Can you work these out from the model? Positions are in its coordinate system, mm. A direction names the side the tool comes from. Coordinates: 2 decimals unless noted, no trailing zeros. Write each loop counter-clockwise with the first axis right and the second up, starting at its lowest first coordinate (ties: lowest second). Pieces come first, ordered by that corner, then holes. Notation, with made-up numbers: (37, 17) - (86, 17) arc R13 cw to (86, 22) - close; hole circle Ø11 at (-23.5, -5.75). An arc over 180 degrees is marked (long way). Write each question's results on one line, items separated by ' | '. Start each with the question number.
```python
from build123d import *

# Parameters (mm, degrees)
SKETCH1_W              = 25
SKETCH1_H              = 25
SKETCH1_R              = 9.5
ALONGSIDE_WASHER_DEPTH = 2
SKETCH2_W              = 25
SKETCH2_H              = 25
BELOW_WASHER_DEPTH     = 1
SKETCH3_W              = 5
SKETCH3_H              = 25
UPRIGHT_1_DEPTH        = 15.6
SKETCH4_W              = 25
SKETCH4_H              = 1.2
BOSS_EXTRUDE4_DEPTH    = 25
SKETCH5_R              = 2.75
CUT_EXTRUDE1_DEPTH     = 1.2
BOSS_EXTRUDE5_START    = -1.2
SKETCH6_W              = 25
SKETCH6_H              = 25
BOSS_EXTRUDE5_DEPTH    = 6.2
SKETCH7_R              = 3.1
CUT_EXTRUDE2_DEPTH     = 40.930063862
SKETCH8_W              = 25
SKETCH8_H              = 4.2
BOSS_EXTRUDE6_DEPTH    = 37
BOSS_EXTRUDE7_START    = -1
SKETCH9_R              = 1
BOSS_EXTRUDE7_DEPTH    = 1


with BuildPart() as part:
    # Sketch1 → alongside washer (new body)
    with BuildSketch(Plane(origin=(0, 0, 0), x_dir=(1, 0, 0), z_dir=(0, 1, 0))):
        Rectangle(SKETCH1_W, SKETCH1_H)
        with Locations(Location((0, 0, 0), (0, 0, 270))):
            Circle(SKETCH1_R, mode=Mode.SUBTRACT)
    extrude(amount=ALONGSIDE_WASHER_DEPTH)

    # Sketch2 → below washer (add)
    with BuildSketch(Plane.XZ):
        Rectangle(SKETCH2_W, SKETCH2_H)
    extrude(amount=BELOW_WASHER_DEPTH)

    # Sketch3 → upright 1 (add)
    with BuildSketch(Plane.XZ.offset(1)):
        with Locations((-15, 0)):
            Rectangle(SKETCH3_W, SKETCH3_H)
    upright_1 = extrude(amount=-UPRIGHT_1_DEPTH)

    # Sketch4 → Boss-Extrude4 (add)
    with BuildSketch(Plane(origin=(-12.5, 0, 0), x_dir=(0, 0, -1), z_dir=(1, 0, 0))):
        with Locations((0, 8)):
            Rectangle(SKETCH4_W, SKETCH4_H)
    extrude(amount=BOSS_EXTRUDE4_DEPTH)

    # Sketch5 → Cut-Extrude1 (cut)
    with BuildSketch(Plane(origin=(0, 8.6, 0), x_dir=(1, 0, 0), z_dir=(0, 1, 0))):
        with Locations(Location((0, 0, 0), (0, 0, 270))):
            Circle(SKETCH5_R)
    extrude(amount=-CUT_EXTRUDE1_DEPTH, mode=Mode.SUBTRACT)

    # Sketch6 → Boss-Extrude5 (add)
    with BuildSketch(Plane(origin=(0, 8.6, 0), x_dir=(1, 0, 0), z_dir=(0, 1, 0)).offset(BOSS_EXTRUDE5_START)):
        Rectangle(SKETCH6_W, SKETCH6_H)
        Polygon((3.9, 2.25166605), (0, 4.5033321), (-3.9, 2.25166605), (-3.9, -2.25166605), (0, -4.5033321), (3.9, -2.25166605), align=None, mode=Mode.SUBTRACT)
    extrude(amount=BOSS_EXTRUDE5_DEPTH)

    # Mirror1: upright 1 across plane
    add(upright_1.mirror(Plane(origin=(0, 0, 0), x_dir=(0, 0, 1), z_dir=(1, 0, 0))))

    # Sketch7 → Cut-Extrude2 (cut, through all)
    with BuildSketch(Plane(origin=(17.5, 0, 0), x_dir=(0, 0, -1), z_dir=(1, 0, 0))):
        with Locations((0, 5.2)):
            Circle(SKETCH7_R)
    extrude(amount=-CUT_EXTRUDE2_DEPTH, mode=Mode.SUBTRACT)

    # Sketch8 → Boss-Extrude6 (add)
    with BuildSketch(Plane(origin=(12.5, 0, 0), x_dir=(0, 0, -1), z_dir=(1, 0, 0))):
        with Locations((0, 12.5)):
            Rectangle(SKETCH8_W, SKETCH8_H)
    extrude(amount=BOSS_EXTRUDE6_DEPTH)

    # Sketch9 → Boss-Extrude7 (add)
    with BuildSketch(Plane.ZY.offset(-12.5).offset(BOSS_EXTRUDE7_START)):
        with BuildLine():
            ThreePointArc((-2.184032967, 7.4), (-1.191532166, 2.338138526), (3.1, 5.2))
            ThreePointArc((3.1, 5.2), (2.861861474, 6.391532166), (2.184032967, 7.4))
            ThreePointArc((2.184032967, 7.4), (0, 8.3), (-2.184032967, 7.4))
        make_face()
        with Locations((0, 5.2)):
            Circle(SKETCH9_R, mode=Mode.SUBTRACT)
    extrude(amount=BOSS_EXTRUDE7_DEPTH)


solid = part.part
```
Q1. If we section it at C-C (z = 0): Count the separate pieces of the cut face and the enclosed holes in it, then the cut area to 3 significant figures.
Q2. I need wall thicknesses on line 1 along X through (y, z) = (2.25, 2.75); line 2 along Y through (x, z) = (-9, -8); line 3 along Y through (x, z) = (-5.5, 0). Which ranges of each line are inside material? Lowest first, please. Write a range as from..to.
Q3. Thinking about a two-plate mould opening in X: for faces 1 (the face through (13.5, 6, -1)), 2 (the face through (-9, 2, -6)), 3 (the face through (15.528, 4.013, -2.864)), which applies, pulls with the +X half, pulls with the -X half, needs draft (parallel to the pull), parting line crosses it, or undercut?
Q4. If we section it at B-B (x = -7.5): Please give me the cut outline in (y, z).
Q5. For faces 4 (the face through (1.98, 11.06, -3.36)), 5 (the face through (-12.5, 3, -3)), 6 (the face through (17.5, 3, -3)), 7 (the face through (0, 0, 0)), which set-ups out of +Z, -Z, +X, -X, +Y, -Y let a thin tool reach every point of the face, with its end or its side?
Q6. If we section it at A-A (y = 5.2): Please give me the cut outline in (x, z), then the cut area to 3 significant figures.
Q7. I'm going to push flat-ended pins straight in: pin 1 Ø12.5 at (x, z) = (4, 5.5) entering from +Y; pin 2 Ø3 at (y, z) = (4, 1.5) entering from +X; pin 3 Ø3 at (y, z) = (5.2, 0) entering from -X. Where does each tip first touch, or does it pass through?
Q8. If we section it at D-D (z = -7): Please give me the cut outline in (x, y), then the cut area to 3 significant figures.
Answer list:
1) separate pieces: 3 | enclosed holes: 0 | area: 361 mm2
2) line 1: x = -17.5..-12.5, 12.5..17.5 | line 2: y = -1..2, 7.4..13.6 | line 3: y = -1..0, 8.3..13.6
3) face 1: pulls with the +X half | face 2: undercut | face 3: needs draft
4) outline: (-1, -12.5) - (2, -12.5) - (2, -5.83) - (0, -5.83) - (0, 5.83) - (2, 5.83) - (2, 12.5) - (-1, 12.5) - close; (7.4, -12.5) - (13.6, -12.5) - (13.6, 12.5) - (7.4, 12.5) - (7.4, 2.18) arc R3.1 cw to (7.4, -2.18) - close
5) face 4: +Y | face 5: +Z, -Z | face 6: +Z, -Z, +X, -Y | face 7: none
6) outline: (-17.5, -12.5) - (-12.5, -12.5) - (-12.5, -3.1) - (-17.5, -3.1) - close; (-17.5, 3.1) - (-12.5, 3.1) - (-12.5, 12.5) - (-17.5, 12.5) - close; (12.5, -12.5) - (17.5, -12.5) - (17.5, -3.1) - (13.5, -3.1) - (13.5, -1) - (12.5, -1) - close; (12.5, 1) - (13.5, 1) - (13.5, 3.1) - (17.5, 3.1) - (17.5, 12.5) - (12.5, 12.5) - close | area: 192 mm2
7) pin 1: stops at y = 13.6 | pin 2: stops at x = 17.5 | pin 3: stops at x = 12.5
8) outline: (-17.5, -1) - (17.5, -1) - (17.5, 10.4) - (49.5, 10.4) - (49.5, 14.6) - (12.5, 14.6) - (12.5, 13.6) - (-12.5, 13.6) - (-12.5, 14.6) - (-17.5, 14.6) - close; hole (-12.5, 2) - (-6.42, 2) - (-6.42, 0) - (6.42, 0) - (6.42, 2) - (12.5, 2) - (12.5, 7.4) - (-12.5, 7.4) - close | area: 495 mm2
